Input: part model. Units: mm. Frame: model coordinates. A direction names the side the tool comes from. Round coordinates to 2 decimals unless told otherwise and drop trailing zeros. Order: outer loops, then holes, each group sorted by start corner. A loop starts at its lowest first (then second) coordinate and runs counter-clockwise, first axis right, second up. Notation, with made-up numbers: (63, -33.75) -> (79, -33.75) arc R22 cw to (79, -2.75) -> close; hole circle Ø11 at (48, -30.75). An arc over 180 degrees is marked (long way). Use a Markdown table: item, result.
from build123d import *

# Parameters (mm, degrees)
SKETCH1_R           = 10.5
BOSS_EXTRUDE1_DEPTH = 21
BOSS_EXTRUDE1_TAPER = 1
SKETCH2_R           = 9
CUT_EXTRUDE1_DEPTH  = 20
FILLET1_R           = 1
SKETCH3_W           = 1
SKETCH3_H           = 9.150746373
BOSS_EXTRUDE2_DEPTH = 0.05


with BuildPart() as part:
    # Sketch1 → Boss-Extrude1 (new body)
    with BuildSketch(Plane(origin=(0, 0, 0), x_dir=(1, 0, 0), z_dir=(0, 1, 0))):
        Circle(SKETCH1_R)
    extrude(amount=BOSS_EXTRUDE1_DEPTH, taper=BOSS_EXTRUDE1_TAPER)

    # Sketch2 → Cut-Extrude1 (cut)
    with BuildSketch(Plane.XZ):
        Circle(SKETCH2_R)
    extrude(amount=-CUT_EXTRUDE1_DEPTH, mode=Mode.SUBTRACT)

    # Fillet1
    fillet1_edges = [part.edges().sort_by_distance(p)[0] for p in [
        (-10.133443637, 21, 0),
    ]]
    fillet(fillet1_edges, radius=FILLET1_R)

    # Sketch3 → Boss-Extrude2 (add)
    with BuildSketch(Plane(origin=(0, 21, 0), x_dir=(1, 0, 0), z_dir=(0, 1, 0))):
        with Locations((0, -4.575373187)):
            Rectangle(SKETCH3_W, SKETCH3_H)
    extrude(amount=BOSS_EXTRUDE2_DEPTH)


solid = part.part
1) Cut plane A-A on y = 4.25. Return loops of the section in (x, z), and give its area (3 significant figures).
Results found:
| item | result |
|---|---|
| outline | circle Ø20.85 at (0, 0); hole circle Ø18 at (0, 0) |
| area | 87.0 mm² |
2) Set-up query: faces 4 (the cylindrical face through (-1.172, 9.86, 8.923)), 5 (the flat face through (0, 21.05, 5)). Return all of +Z, -Z, +X, -X, +Y, -Y with unobstructed straight access to the full face (end or side cutting, diameter ignored); none if empty.
Results found:
| item | result |
|---|---|
| face 4 | -Y |
| face 5 | +Z, -Z, +X, -X, +Y |
3) Line query: L1, parallel to Y at x = 3.5, z = 7.75; L2, parallel to Z at x = 0, y = 11; L3, parallel to Z at x = 0, y = 4.25. Output: solid intervals per line, ascending. Write a range as [from, to].
Results found:
| item | result |
|---|---|
| L1 | y = [20, 21] |
| L2 | z = [-10.31, -9], [9, 10.31] |
| L3 | z = [-10.43, -9], [9, 10.43] |
4) Pull-direction query (X, two-part tool) for faces 1 (the conical face through (-10.313, 10.149, -0.454)), 2 (the flat face through (8, 0, -5)), 3 (the flat face through (0, 20, 0)); classes: +X half, -X half, draft (parallel to the pull), parting line (faces both ways), or undercut.
Results found:
| item | result |
|---|---|
| face 1 | parting line |
| face 2 | draft |
| face 3 | undercut |
5) Cut plane B-B on y = 14. Return loops of the section in (x, z).
Results found:
| item | result |
|---|---|
| outline | circle Ø20.51 at (0, 0); hole circle Ø18 at (0, 0) |
6) Pin query (flat end, axial travel): pin 1 Ø2 at (x, z) = (7.5, -5.5) entering from +Y; pin 2 Ø11 at (x, z) = (0, 0) entering from -Y; pin 3 Ø1.5 at (y, z) = (12.5, 2) entering from -X. Return the tip coordinate at first contact, or that it passes through.
Results found:
| item | result |
|---|---|
| pin 1 | stops at y = 21 |
| pin 2 | stops at y = 20 |
| pin 3 | stops at x = -10.21 |
